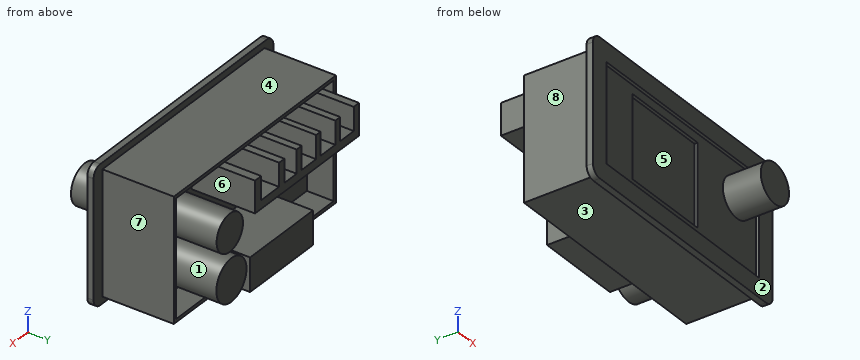
from build123d import *

# Parameters (mm, degrees)
SKETCH1_W           = 79.5
SKETCH1_H           = 43
BOSS_EXTRUDE1_DEPTH = 2
SKETCH2_W           = 71.7
SKETCH2_H           = 38.8
BOSS_EXTRUDE2_DEPTH = 22.6
SKETCH3_W           = 69.7
SKETCH3_H           = 36.8
CUT_EXTRUDE1_DEPTH  = 8.5
BOSS_EXTRUDE3_DEPTH = 22.6
SKETCH6_W           = 67.219676188
SKETCH6_H           = 8.940869551
CUT_EXTRUDE2_DEPTH  = 22.6
SKETCH7_R           = 6.66374012
SKETCH7_R_2         = 5.829163104
BOSS_EXTRUDE4_DEPTH = 20.1
FILLET1_R           = 3
SKETCH8_W           = 27.801535977
SKETCH8_H           = 10.55826339
BOSS_EXTRUDE5_DEPTH = 17
SKETCH9_W           = 67.5
SKETCH9_H           = 31
CUT_EXTRUDE3_DEPTH  = 1
SKETCH10_W          = 28.845725121
SKETCH10_H          = 25.974204973
CUT_EXTRUDE4_DEPTH  = 1
SKETCH11_R          = 6.25
BOSS_EXTRUDE6_DEPTH = 12


with BuildPart() as part:
    # Sketch1 → Boss-Extrude1 (new body)
    with BuildSketch(Plane(origin=(0, 0, 0), x_dir=(1, 0, 0), z_dir=(0, 1, 0))):
        with Locations((25.074854651, -17.802325581)):
            Rectangle(SKETCH1_W, SKETCH1_H)
    extrude(amount=BOSS_EXTRUDE1_DEPTH)

    # Sketch2 → Boss-Extrude2 (add)
    with BuildSketch(Plane(origin=(0, 2, 0), x_dir=(1, 0, 0), z_dir=(0, 1, 0))):
        with Locations((25.074854651, -17.802325581)):
            Rectangle(SKETCH2_W, SKETCH2_H)
    extrude(amount=BOSS_EXTRUDE2_DEPTH)

    # Sketch3 → Cut-Extrude1 (cut)
    with BuildSketch(Plane(origin=(0, 24.6, 0), x_dir=(1, 0, 0), z_dir=(0, 1, 0))):
        with Locations((25.074854651, -17.802325581)):
            Rectangle(SKETCH3_W, SKETCH3_H)
    extrude(amount=-CUT_EXTRUDE1_DEPTH, mode=Mode.SUBTRACT)

    # Sketch5 → Boss-Extrude3 (add)
    with BuildSketch(Plane(origin=(0, 16.1, 0), x_dir=(1, 0, 0), z_dir=(0, 1, 0))):
        Polygon((41.224854651, -26.202325581), (-4.775145349, -26.202325581), (-4.775145349, -36.202325581), (-2.433003128, -36.202325581), (-2.433003128, -28.831573422), (3.571084453, -28.831573422), (3.571084453, -36.202325581), (5.724724564, -36.202325581), (5.724724564, -28.831573422), (12.250906718, -28.831573422), (12.250906718, -36.202325581), (14.208761365, -36.202325581), (14.208761365, -28.831573422), (20.604419876, -28.831573422), (20.604419876, -36.202325581), (22.823321808, -36.202325581), (22.823321808, -28.831573422), (28.240052996, -28.831573422), (28.240052996, -36.202325581), (30.589478571, -36.202325581), (30.589478571, -28.831573422), (38.486158978, -28.831573422), (38.486158978, -36.202325581), (41.224854651, -36.202325581), align=None)
    extrude(amount=BOSS_EXTRUDE3_DEPTH)

    # Sketch6 → Cut-Extrude2 (cut)
    with BuildSketch(Plane.XY.offset(37.202325581)):
        with Locations((18.972874337, 40.670434775)):
            Rectangle(SKETCH6_W, SKETCH6_H)
    extrude(amount=-CUT_EXTRUDE2_DEPTH, mode=Mode.SUBTRACT)

    # Sketch7 → Boss-Extrude4 (add)
    with BuildSketch(Plane(origin=(0, 16.1, 0), x_dir=(1, 0, 0), z_dir=(0, 1, 0))):
        with Locations((51.669046929, -11.341405249)):
            Circle(SKETCH7_R)
        with Locations((52.386926966, -26.090576917)):
            Circle(SKETCH7_R_2)
    extrude(amount=BOSS_EXTRUDE4_DEPTH)

    # Fillet1
    fillet1_edges = [part.edges().sort_by_distance(p)[0] for p in [
        (-14.675145349, 1, -3.697674419),
        (64.824854651, 1, -3.697674419),
        (64.824854651, 1, 39.302325581),
        (-14.675145349, 1, 39.302325581),
    ]]
    fillet(fillet1_edges, radius=FILLET1_R)

    # Sketch8 → Boss-Extrude5 (add)
    with BuildSketch(Plane(origin=(0, 16.1, 0), x_dir=(1, 0, 0), z_dir=(0, 1, 0))):
        with Locations((25.172747384, -5.279131695)):
            Rectangle(SKETCH8_W, SKETCH8_H)
    extrude(amount=BOSS_EXTRUDE5_DEPTH)

    # Sketch9 → Cut-Extrude3 (cut)
    with BuildSketch(Plane.XZ):
        with Locations((25.074854651, 17.802325581)):
            Rectangle(SKETCH9_W, SKETCH9_H)
    extrude(amount=-CUT_EXTRUDE3_DEPTH, mode=Mode.SUBTRACT)

    # Sketch10 → Cut-Extrude4 (cut)
    with BuildSketch(Plane.XZ.offset(-1)):
        with Locations((18.581303408, 17.606540116)):
            Rectangle(SKETCH10_W, SKETCH10_H)
    extrude(amount=-CUT_EXTRUDE4_DEPTH, mode=Mode.SUBTRACT)

    # Sketch11 → Boss-Extrude6 (add)
    with BuildSketch(Plane.XZ.offset(-1)):
        with Locations((50.42907232, 22.696962197)):
            Circle(SKETCH11_R)
    extrude(amount=BOSS_EXTRUDE6_DEPTH)


solid = part.part
Design review of the part built by this model. Coordinates are the model's own, in mm. Face numbers are marked on the shaded views. A direction names the side the tool comes from. Round coordinates to 2 decimals unless told otherwise and drop trailing zeros. Write each loop counter-clockwise with the first axis right and the second up, starting at its lowest first coordinate (ties: lowest second). Pieces come first, ordered by that corner, then holes. Notation, with made-up numbers: M 5.5,87 L 53.5,87 A17 cw 53.5,108 Z; hole C 7,39.5 d5. An arc over 180 degrees is marked long. One line per item, written item: value. Start each with the question number.
1. Take a section at A-A on y = 30.5. State how many separate pieces and enclosed holes the cut face has, then the cut area to 3 significant figures.
2. To check wall thickness, follow probe 1 along Z at (x, y) = (17.5, 20); probe 2 along X at (y, z) = (1.5, 26); probe 3 along X at (y, z) = (23, 23.5). State the ranges of each line that lie inside material, in increasing order. Write a range as from..to.
3. Take a section at D-D on z = 9.5. State the section outline as (x, y) points, then the cut area to 3 significant figures.
4. For the marked faces 4, 5, 6, 7 and 8, list the 3-axis set-ups (+Z, -Z, +X, -X, +Y, -Y) from which the entire face can be reached by the end or side of a thin tool; tool diameter is ignored.
5. Draft analysis for pull direction Z (two halves, no side actions). For the marked faces 1, 2 and 3, state which applies: pulls with the +Z half, pulls with the -Z half, needs draft (parallel to the pull), parting line crosses it, or undercut.
6. Clearance check with flat-ended pins moving along their axes: P1, Ø1, axis at x = 13.5, y = 29, coming from the +Z side; P2, Ø7, axis at x = 17.5, y = 22.5, coming from the -Z side; P3, Ø8, axis at y = 17.5, z = 26, coming from the -X side; P4, Ø6, axis at x = 26, z = 31, coming from the +Y side. State where each tip first meets the part, or that it passes through.
7. Take a section at B-B on x = 34. State the section outline as (y, z) points, then the cut area to 3 significant figures.
Computed:
1. separate pieces: 4
1. enclosed holes: 0
1. area: 762 mm²
2. probe 1: z = -1.6..-0.6, 0..10.56, 26.2..28.83, 36.2..37.2
2. probe 2: x = -14.68..4.16, 33..64.82
2. probe 3: x = -10.78..-9.78, 47.17..57.61, 59.92..60.92
3. outline: M -14.68,0 L -8.68,0 L -8.68,1 L 4.16,1 L 4.16,2 L 33,2 L 33,1 L 58.82,1 L 58.82,0 L 64.82,0 L 64.82,2 L 60.92,2 L 60.92,24.6 L 59.92,24.6 L 59.92,16.1 L 58.07,16.1 L 58.07,36.2 L 45.26,36.2 L 45.26,16.1 L 39.07,16.1 L 39.07,33.1 L 11.27,33.1 L 11.27,16.1 L -9.78,16.1 L -9.78,24.6 L -10.78,24.6 L -10.78,2 L -14.68,2 Z
3. area: 1,820 mm²
4. face 4: +Z, +X, -X, +Y
4. face 5: -Y
4. face 6: +Y
4. face 7: +Z, -Z, +X, +Y
4. face 8: +Z, -Z, -X, +Y
5. face 1: undercut
5. face 2: needs draft
5. face 3: pulls with the -Z half
6. P1: stops at z = 36.2
6. P2: stops at z = -1.6
6. P3: stops at x = -10.78
6. P4: stops at y = 36.2
7. outline: M 0,-3.7 L 2,-3.7 L 2,-1.6 L 24.6,-1.6 L 24.6,-0.6 L 16.1,-0.6 L 16.1,0 L 33.1,0 L 33.1,10.56 L 16.1,10.56 L 16.1,26.2 L 36.2,26.2 L 36.2,28.83 L 16.1,28.83 L 16.1,36.2 L 24.6,36.2 L 24.6,37.2 L 2,37.2 L 2,39.3 L 0,39.3 L 0,33.3 L 1,33.3 L 1,2.3 L 0,2.3 Z
7. area: 851 mm²
